Work out the finished part from the listing and answer in its coordinate system (mm). Face numbers are marked on the shaded views. Round coordinates to 2 decimals unless told otherwise and drop trailing zeros. Loops run counter-clockwise (first coordinate to the right, second up) from the corner with the lowest first, then second, coordinate; pieces in that order, holes last.
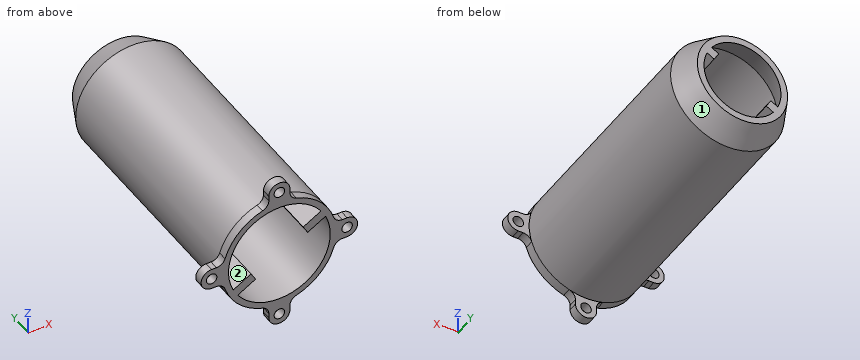
```python
from build123d import *
from build123d.topology import SkipClean

# Parameters (mm, degrees)
SKETCH2_R           = 1.75
CUT_EXTRUDE1_DEPTH  = 10
SKETCH4_R           = 36.837485066
SKETCH4_R_2         = 31.9
CUT_EXTRUDE2_DEPTH  = 99.001122443
FILLET1_R           = 3
BOSS_EXTRUDE1_REACH = 99.221


with BuildPart() as part:
    # Sketch1 → Revolve1 (revolve)
    with BuildSketch(Plane(origin=(0, 0, 0), x_dir=(0, 0, -1), z_dir=(1, 0, 0)), mode=Mode.PRIVATE) as revolve1_sk:
        Polygon((-12.793244162, 90), (-15, 90), (-18.9, 81.63642301), (-18.9, 3), (-31.9, 3), (-31.9, 0), (-17.6, 0), (-16.9, 0), (-16.9, 81.193033685), align=None)
    revolve(revolve1_sk.sketch.rotate(Axis((0, -1110.96911415, 0), (0, 1, 0)), 180), axis=Axis((0, -1110.96911415, 0), (0, 1, 0)))

    # Sketch2 → Cut-Extrude1 (cut)
    with BuildSketch(Plane.XZ):
        with Locations(Location((0, 22.5, 0), (0, 0, 270))):
            Circle(SKETCH2_R)
        with Locations(Location((0, -22.5, 0), (0, 0, 270))):
            Circle(SKETCH2_R)
        with Locations(Location((-22.5, 0, 0), (0, 0, 270))):
            Circle(SKETCH2_R)
        with Locations(Location((22.5, 0, 0), (0, 0, 270))):
            Circle(SKETCH2_R)
    extrude(amount=-CUT_EXTRUDE1_DEPTH, mode=Mode.SUBTRACT)

    # Sketch4 → Cut-Extrude2 (cut, through all)
    # profile 1 of 2: a face of its own
    with SkipClean():  # the faces are left unmerged after this step: merging them gives an invalid solid
        with BuildSketch(Plane(origin=(0, 3, 0), x_dir=(1, 0, 0), z_dir=(0, 1, 0))):
            Circle(SKETCH4_R)
            Circle(SKETCH4_R_2, mode=Mode.SUBTRACT)
        # profile 2 of 2: a face of its own
        with BuildSketch(Plane(origin=(0, 3, 0), x_dir=(1, 0, 0), z_dir=(0, 1, 0))):
            Circle(SKETCH4_R_2)
            with BuildLine():
                Line((-3.5, 18.573098826), (-3.5, 22.5))
                ThreePointArc((-3.5, 22.5), (0, 26), (3.5, 22.5))
                Line((3.5, 22.5), (3.5, 18.573098826))
                ThreePointArc((3.5, 18.573098826), (13.364318164, 13.364318164), (18.573098826, 3.5))
                Line((18.573098826, 3.5), (22.5, 3.5))
                ThreePointArc((22.5, 3.5), (26, 0), (22.5, -3.5))
                Line((22.5, -3.5), (18.573098826, -3.5))
                ThreePointArc((18.573098826, -3.5), (13.364318164, -13.364318164), (3.5, -18.573098826))
                Line((3.5, -18.573098826), (3.5, -22.5))
                ThreePointArc((3.5, -22.5), (0, -26), (-3.5, -22.5))
                Line((-3.5, -22.5), (-3.5, -18.573098826))
                ThreePointArc((-3.5, -18.573098826), (-13.364318164, -13.364318164), (-18.573098826, -3.5))
                Line((-18.573098826, -3.5), (-22.5, -3.5))
                ThreePointArc((-22.5, -3.5), (-26, 0), (-22.5, 3.5))
                Line((-22.5, 3.5), (-18.573098826, 3.5))
                ThreePointArc((-18.573098826, 3.5), (-13.364318164, 13.364318164), (-3.5, 18.573098826))
            make_face(mode=Mode.SUBTRACT)
        extrude(amount=-CUT_EXTRUDE2_DEPTH, mode=Mode.SUBTRACT)

    # Fillet1
    # the kernel refuses this fillet: 3 mm, written as the material it adds along each edge
    with BuildSketch(Plane(origin=(-3.5, 3, -18.573098826), x_dir=(-0.9704272072576611, 0, 0.24139394237241404), z_dir=(0, -1, 0)), Plane(origin=(-18.573098826, 3, 3.5), x_dir=(0.24139394237237982, -3.328806956187132e-15, 0.9704272072576697), z_dir=(0, -1, 0)), Plane(origin=(3.5, 3, 18.573098826), x_dir=(0.970427207257667, 0, -0.24139394237239048), z_dir=(0, -1, 0)), Plane(origin=(18.573098826, 3, -3.5), x_dir=(-0.24139394237243622, 3.3288069561870833e-15, -0.9704272072576556), z_dir=(0, -1, 0))) as fillet1_piece_1:
        with BuildLine():
            CenterArc((2.346406537, 2.995034797), FILLET1_R, 193.968826574, 72.734276137)
            Line((-0.564875085, 2.27085297), (0, 0))
            ThreePointArc((0, 0), (1.086938322, 0.031280778), (2.173876645, 0))
        make_face()
    extrude(amount=3)
    with BuildSketch(Plane(origin=(-18.573098826, 3, -3.5), x_dir=(0.24139394237239928, 3.3288069561871153e-15, -0.9704272072576648), z_dir=(0, -1, 0)), Plane(origin=(-3.5, 3, 18.573098826), x_dir=(-0.9704272072576595, 0, -0.24139394237242057), z_dir=(0, -1, 0)), Plane(origin=(18.573098826, 3, 3.5), x_dir=(-0.24139394237244305, -3.328806956187078e-15, 0.970427207257654), z_dir=(0, -1, 0)), Plane(origin=(3.5, 3, -18.573098826), x_dir=(0.9704272072576657, 0, 0.2413939423723955), z_dir=(0, -1, 0))) as fillet1_piece_2:
        with BuildLine():
            CenterArc((2.346406537, -2.995034797), FILLET1_R, 93.296897289, 72.734276137)
            Line((-0.564875085, -2.27085297), (0, 0))
            ThreePointArc((0, 0), (1.086938322, -0.031280778), (2.173876645, 0))
        make_face()
    extrude(amount=3)

    # Boss-Extrude1: up to this cone (the profile starts inside it)
    boss_extrude1_end = Plane(origin=(0, 0, 0), z_dir=(0, -1, 0)).offset(-117.435199641) * Cone(1e-06, 126.797041985, 271.917133037, align=(Align.CENTER, Align.CENTER, Align.MIN), mode=Mode.PRIVATE)
    # Sketch5 → Boss-Extrude1 (add, up to the surface)
    with BuildSketch(Plane.XZ, mode=Mode.PRIVATE) as boss_extrude1_sk1:
        Polygon((14.838457268, 10.299038106), (16.338457268, 7.700961894), (9.410254038, 3.700961894), (7.910254038, 6.299038106), align=None)
    boss_extrude1_tool1 = extrude(boss_extrude1_sk1.sketch, amount=-BOSS_EXTRUDE1_REACH, mode=Mode.PRIVATE) & boss_extrude1_end
    add(boss_extrude1_tool1.solids().sort_by_distance((12.124356, 0, 7))[0])
    # Sketch5 → Boss-Extrude1 (add, up to the surface)
    with BuildSketch(Plane.XZ, mode=Mode.PRIVATE) as boss_extrude1_sk2:
        Polygon((-14.838457268, -10.299038106), (-16.338457268, -7.700961894), (-9.410254038, -3.700961894), (-7.910254038, -6.299038106), align=None)
    boss_extrude1_tool2 = extrude(boss_extrude1_sk2.sketch, amount=-BOSS_EXTRUDE1_REACH, mode=Mode.PRIVATE) & boss_extrude1_end
    add(boss_extrude1_tool2.solids().sort_by_distance((-12.124356, 0, -7))[0])

    # SurfaceCut2
    split(bisect_by=Plane(origin=(0, 90, 0), x_dir=(1, 0, 0), z_dir=(0, 1, 0)), keep=Keep.BOTTOM)


solid = part.part
```
1. Determine the mould class of the marked faces 1 and 2 for opening direction X: +X half, -X half, draft (parallel to the pull), parting line (faces both ways), or undercut.
Answer key:
face 1: parting line
face 2: undercut
2. Find section A-A (y = 32.5). Write down the section's boundary in (x, z).
Answer key:
outline: circle Ø37.8 at (0, 0); hole (-15.33, -7.12) - (-9.41, -3.7) - (-7.91, -6.3) - (-13.83, -9.72) arc R16.9 ccw to (15.33, 7.12) - (9.41, 3.7) - (7.91, 6.3) - (13.83, 9.72) arc R16.9 ccw to start
3. Find section C-C (z = 0). Write down the section's boundary in (x, y).
Answer key:
outline: (-26, 0) - (-24.25, 0) - (-24.25, 3) - (-26, 3) - close; (-20.75, 0) - (-16.9, 0) - (-16.9, 81.19) - (-12.79, 90) - (-15, 90) - (-18.9, 81.64) - (-18.9, 3) - (-20.75, 3) - close; (12.79, 90) - (16.9, 81.19) - (16.9, 0) - (20.75, 0) - (20.75, 3) - (18.9, 3) - (18.9, 81.64) - (15, 90) - close; (24.25, 0) - (26, 0) - (26, 3) - (24.25, 3) - close
4. Find section D-D (y = 83). Write down the section's boundary in (x, z), then the cut area to 3 significant figures.
Answer key:
outline: circle Ø36.53 at (0, 0); hole (-14.6, -6.69) - (-9.41, -3.7) - (-7.91, -6.3) - (-13.1, -9.29) arc R16.06 ccw to (14.6, 6.69) - (9.41, 3.7) - (7.91, 6.3) - (13.1, 9.29) arc R16.06 ccw to start
area: 274 mm2
5. Find section B-B (x = 0). Write down the section's boundary in (y, z).
Answer key:
outline: (0, -26) - (3, -26) - (3, -24.25) - (0, -24.25) - close; (0, -20.75) - (3, -20.75) - (3, -18.9) - (81.64, -18.9) - (90, -15) - (90, -12.79) - (81.19, -16.9) - (0, -16.9) - close; (0, 16.9) - (81.19, 16.9) - (90, 12.79) - (90, 15) - (81.64, 18.9) - (3, 18.9) - (3, 20.75) - (0, 20.75) - close; (0, 24.25) - (3, 24.25) - (3, 26) - (0, 26) - close
6. Given pin 1 (1.3 mm diameter, centred on x = -21.5, y = 1, fed in from +Z); pin 2 (2.5 mm diameter, centred on x = -0.5, z = 22, fed in from +Y); pin 3 (0.8 mm diameter, centred on x = 22, y = 2, fed in from -Z); pin 4 (2 mm diameter, centred on x = 22.5, z = 0, fed in from -Y), each flat-ended and moving along its own axis, determine where each tip first touches the part or whether it passes through.
Answer key:
pin 1: stops at z = 3.5
pin 2: stops at y = 3
pin 3: stops at z = -3.5
pin 4: passes through
7. Consider probe 1 along X at (y, z) = (0.7, 22.5); probe 2 along X at (y, z) = (66, 6.5); probe 3 along X at (y, z) = (85, -12.5). Determine where each line is inside the solid, lowest interval first.
Answer key:
probe 1: x = -3.5 to -1.75, 1.75 to 3.5
probe 2: x = -17.75 to -15.6, 8.26 to 14.26, 15.6 to 17.75
probe 3: x = -12.01 to -8.52, 8.52 to 12.01
